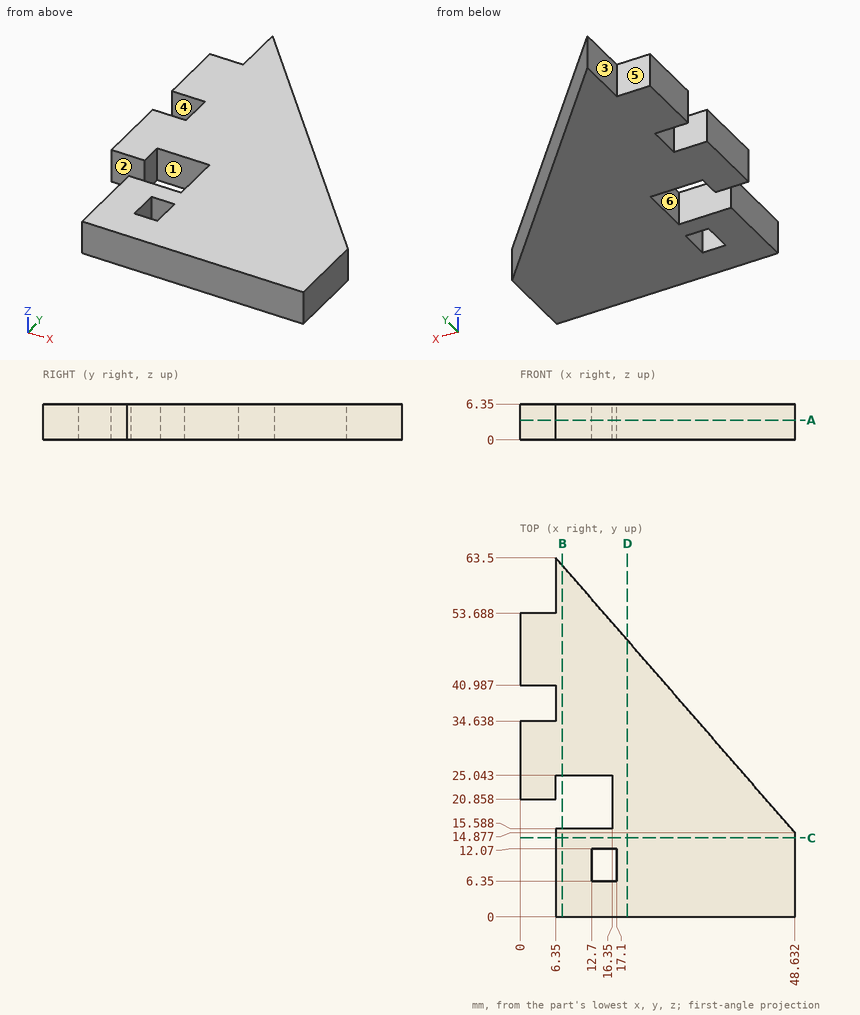
Study the drawing (mm; zero at the part's minimum x, y, z) and answer. A direction names the side the tool comes from. Coordinates: 2 decimals unless noted, no trailing zeros. Loops run counter-clockwise (first coordinate to the right, second up) from the corner with the lowest first, then second, coordinate; pieces in that order, holes last. Notation, with made-up numbers: (15, 2) -> (28, 2) arc R11 cw to (28, 7) -> close; hole circle Ø3 at (56.25, 13). An arc over 180 degrees is marked (long way). Write item = value, one per line. Start each with the question number.
1) The part is cut by section B-B, the plane x = 7.5. Determine the outline of the cut face in (y, z).
2) For the marked faces 4, 5 and 6, determine the directions among +Z, -Z, +X, -X, +Y, -Y from which every point of the face is accessible in a straight line to the end or side of a thin tool.
3) The part is cut by section D-D, the plane x = 19. Determine the outline of the cut face in (y, z).
4) Given P1, Ø1.9, axis at y = 7, z = 4.5, coming from the -X side; P2, Ø2, axis at x = 16, z = 2.5, coming from the -Y side; P3, Ø1.3, axis at y = 22.5, z = 4.5, coming from the +X side; P4, Ø1.9, axis at x = 12, z = 2, coming from the +Y side (1 decimal), each flat-ended and moving along its own axis, determine where each tip first touches the part or whether it passes through.
5) The part is cut by section C-C, the plane y = 14. Determine the outline of the cut face in (x, z).
6) The mould has two halves that part along Y. Classify the marked faces 1, 2 and 3: pulls with the +Y half, pulls with the -Y half, needs draft (parallel to the pull), parting line crosses it, or undercut.
7) Find the intervals of material crossed by L1, parallel to Y at x = 2, z = 6; L2, parallel to X at y = 3, z = 3.5; L3, parallel to Y at x = 8.5, z = 5 (1 decimal), in increasing order. Write a range as from..to.
8) The part is cut by section A-A, the plane z = 3.5. Determine the outline of the cut face in (x, y).
Result:
q1.outline = (0, 0) -> (15.59, 0) -> (15.59, 6.35) -> (0, 6.35) -> close; (25.04, 0) -> (62.18, 0) -> (62.18, 6.35) -> (25.04, 6.35) -> close
q2.face_4 = +Z, -Z, -X
q2.face_5 = +Z, -Z, -X, +Y
q2.face_6 = +Z, -Z
q3.outline = (0, 0) -> (48.95, 0) -> (48.95, 6.35) -> (0, 6.35) -> close
q4.P1 = 6.35
q4.P2 = 0
q4.P3 = 42.57
q4.P4 = 58.1
q5.outline = (6.35, 0) -> (48.63, 0) -> (48.63, 6.35) -> (6.35, 6.35) -> close
q6.face_1 = undercut
q6.face_2 = pulls with the -Y half
q6.face_3 = needs draft
q7.L1 = 20.86..34.64, 40.99..53.69
q7.L2 = 6.35..48.63
q7.L3 = 0..15.6, 25..61
q8.outline = (0, 20.86) -> (6.35, 20.86) -> (6.35, 25.04) -> (16.35, 25.04) -> (16.35, 15.59) -> (6.35, 15.59) -> (6.35, 0) -> (48.63, 0) -> (48.63, 14.88) -> (6.35, 63.5) -> (6.35, 53.69) -> (0, 53.69) -> (0, 40.99) -> (6.35, 40.99) -> (6.35, 34.64) -> (0, 34.64) -> close; hole (12.7, 6.35) -> (17.1, 6.35) -> (17.1, 12.07) -> (12.7, 12.07) -> close
